from build123d import *

# Parameters (mm, degrees)
SKETCH2_OUTSIDE_W  = 41.962
SKETCH2_OUTSIDE_H  = 41.962
CUT_EXTRUDE1_DEPTH = 37.599869445
CHAMFER1_SIZE      = 1


with BuildPart() as part:
    # Sketch1 → Revolve1 (revolve)
    with BuildSketch(Plane.XY, mode=Mode.PRIVATE) as revolve1_sk:
        with BuildLine():
            Line((0, 30), (-5, 30))
            ThreePointArc((-5, 30), (-8.987504197, 25.684072353), (-4.370118592, 22.049905139))
            Line((-4.370118592, 22.049905139), (-14.824817763, 5))
            Line((-14.824817763, 5), (-7.627118644, 5))
            Line((-7.627118644, 5), (-7.627118644, 0))
            Line((-7.627118644, 0), (0, 0))
            Line((0, 0), (0, 30))
        make_face()
    revolve(revolve1_sk.sketch.rotate(Axis((0, 0, 0), (0, 1, 0)), 270), axis=Axis((0, 0, 0), (0, 1, 0)))

    # Sketch2 outside → Cut-Extrude1 (cut, through all)
    with BuildSketch(Plane(origin=(0, 30, 0), x_dir=(1, 0, 0), z_dir=(0, 1, 0))):
        Rectangle(SKETCH2_OUTSIDE_W, SKETCH2_OUTSIDE_H)
        Polygon((-12.927457346, -7.256450114), (-0.179458533, -14.823731525), (12.747998813, -7.567281411), (12.927457346, 7.256450114), (0.179458533, 14.823731525), (-12.747998813, 7.567281411), align=None, mode=Mode.SUBTRACT)
    extrude(amount=-CUT_EXTRUDE1_DEPTH, mode=Mode.SUBTRACT)

    # Chamfer1
    chamfer1_edges = [part.edges().sort_by_distance(p)[0] for p in [
        (0, 0, 7.627118644),
    ]]
    chamfer(chamfer1_edges, length=CHAMFER1_SIZE)


solid = part.part
The listing builds one solid part. Answer for the finished solid, in the listing's coordinates (mm). A direction names the side the tool comes from. Give positions to 0.01 mm unless a question says otherwise; leave off trailing zeros. Order: outer loops, then holes, each group sorted by start corner. A loop starts at its lowest first (then second) coordinate and runs counter-clockwise, first axis right, second up. Notation, with made-up numbers: (64.5, 64.5) - (123.5, 64.5) arc R13 cw to (123.5, 70.5) - close; hole circle Ø2 at (47, -17). An arc over 180 degrees is marked (long way). Use one line per item in the form item = value.
1) Consider probe 1 along Z at (x, y) = (-1, 1.5); probe 2 along Y at (x, z) = (3.25, -4.25); probe 3 along Z at (x, y) = (1.75, 18). Determine where each line is inside the solid, lowest interval first. Write a range as [from, to].
Verdict:
probe_1 = [-7.56, 7.56]
probe_2 = [0, 20.45], [22.02, 29.98]
probe_3 = [-6.63, 6.63]
2) Each of these flat-tipped pins is pushed along its axis until it touches: pin 1 (5 mm diameter, centred on y = 12.5, z = -2.5, fed in from -X); pin 2 (12 mm diameter, centred on x = -0.5, y = 17, fed in from -Z); pin 3 (5 mm diameter, centred on x = -9.5, y = 16.5, fed in from +Z). Where does it stop, or does it pass through?
Verdict:
pin_1 = -11.56
pin_2 = -11.14
pin_3 = 4.4
3) For faces 4 (the flat face through (6.64, 6.28, -10.99)), 5 (the cylindrical face through (4.641, 2.972, 6.053)), determine the directions among +Z, -Z, +X, -X, +Y, -Y from which every point of the face is accessible in a straight line to the end or side of a thin tool.
Verdict:
face_4 = -Z, +X, +Y, -Y
face_5 = -Y
4) Find section A-A on z = 0. Determine the outline of the cut face in (x, y).
Verdict:
outline = (-12.84, 5) - (-7.63, 5) - (-7.63, 1) - (-6.63, 0) - (6.63, 0) - (7.63, 1) - (7.63, 5) - (12.84, 5) - (12.84, 8.24) - (4.37, 22.05) arc R4 ccw (long way) to (5, 30) - (-5, 30) arc R4 ccw (long way) to (-4.37, 22.05) - (-12.84, 8.24) - close
5) Find section C-C on y = 14.5. Determine the outline of the cut face in (x, z).
Verdict:
outline = circle Ø18 at (0, 0)
6) Find section B-B on y = 20.5. Determine the outline of the cut face in (x, z).
Verdict:
outline = circle Ø10.64 at (0, 0)
7) The mould has two halves that part along Y. Classify faces 1 (the flat face through (6.19, 6.28, 11.25)), 2 (the flat face through (0, 30, 0)), 3 (the conical face through (5.49, 19.09, -2.85)): released by +Y, released by -Y, zero draft, split by the parting line, or undercut.
Verdict:
face_1 = zero draft
face_2 = released by +Y
face_3 = undercut
